Autodesk Inventor part; units mm, degrees
ref_plane "YZ Plane" through (0, 0, 0) normal (1, 0, 0) x (0, 1, 0)
ref_plane "XZ Plane" through (0, 0, 0) normal (0, 1, 0) x (-1, 0, 0)
ref_plane "XY Plane" through (0, 0, 0) normal (0, 0, 1) x (1, 0, 0)
sketch "Skizze1" plane through (0, 0, 0) normal (0, 0, 1) x (1, 0, 0)
  line L0 (15, -9.5) -> (-15, -9.5)
  line L1 (-15, -9.5) -> (-15, 9.5)
  line L2 (-15, 9.5) -> (15, 9.5)
  line L3 (15, 9.5) -> (15, -9.5)
  line L4 (15, -9.5) -> (-15, 9.5) construction
  line L5 (-15, -9.5) -> (15, 9.5) construction
  point P0 (0, 0)
  dimension "d0" = 30
  dimension "d1" = 19
extrude "Extrusion1" add sketch "Skizze1" along normal blind 22
sketch "Skizze7" plane through (0, 0, 22) normal (0, 0, 1) x (1, 0, 0)
  line L0 (-7.5, -7.5) -> (-7.5, 7.5)
  line L1 (-7.5, 7.5) -> (7.5, 7.5)
  line L2 (7.5, 7.5) -> (7.5, -7.5)
  line L3 (7.5, -7.5) -> (-7.5, -7.5)
  line L4 (15, -9.5) -> (15, 9.5)
  point P0 (0, 0)
  point P1 (0, -7.5)
  point P2 (7.5, 0)
  point P3 (15, 0)
  dimension "d36" = 15
  dimension "d37" = 15
extrude "Extrusion3" add sketch "Skizze7" along normal blind 60
chamfer "Fasen1" distance 2.5 angle 45 2 edges at (-7.5, 7.5, 52) (7.5, 7.5, 52)
sketch "Skizze2" plane through (-15, -9.5, 22) normal (0, 0, 1) x (1, 0, 0)
  line L0 (7, 17.25) -> (23, 17.25)
  line L1 (23, 17.25) -> (23, 1.75)
  line L2 (23, 1.75) -> (7, 1.75)
  line L3 (7, 1.75) -> (7, 17.25)
  line L4 (0, 0) -> (30, 0)
  point P0 (15, 9.5)
  point P1 (15, 1.75)
  point P2 (15, 0)
  point P3 (7, 9.5)
  dimension "d4" = 16
  dimension "d7" = 15.5
extrude "Extrusion2" add sketch "Skizze2" along normal blind 55
sketch "Skizze3" plane through (-15, -9.5, 82) normal (0, 0, 1) x (1, 0, 0)
  line L0 (23, 1.75) -> (23, 17.25)
  line L1 (23, 17.25) -> (7, 17.25)
  point P0 (15, 9.5)
  point P1 (15, 9.5)
  point P2 (23, 9.5)
  point P3 (15, 17.25)
hole "Bohrung1" at (0, 0, 82) direction (0, 0, -1) diameter 2.459 depth 15 tip angle 118
sketch "Skizze4" plane through (-15, -9.5, 0) normal (0, -1, 0) x (1, 0, 0)
  line L0 (0, 0) -> (30, 0)
  line L1 (7, 77) -> (23, 77)
  line L2 (7.5, 82) -> (22.5, 82)
  point P0 (15, 0)
  point P1 (15, 9)
  point P2 (15, 0)
  dimension "d43" = 73
hole "Bohrung2" at (0, -9.5, 9) direction (0, 1, 0) diameter 7.5 depth 9.5 counterbore diameter 10 counterbore depth 4
mirror "Spiegeln1" about plane through (0, 0, 0) normal (0, 1, 0) of "Bohrung2"
sketch "Skizze5" plane through (0, 0, 22) normal (0, 0, 1) x (1, 0, 0)
  circle A0 centre (0, 0) radius 1.2295
  line L0 (15, 9.5) -> (-15, 9.5)
  line L1 (-15, -9.5) -> (15, -9.5)
  point P0 (12, -3)
  point P1 (-12, -3)
  dimension "d30" = 24
  dimension "d31" = 12
  dimension "d34" = 6.5
  dimension "d35" = 6.5
hole "Bohrung3" at (12, -3, 22) at (-12, -3, 22) direction (0, 0, -1) diameter 3.1 depth 22
properties part number "Lagerbock" material "Stahl, galvanisiert"
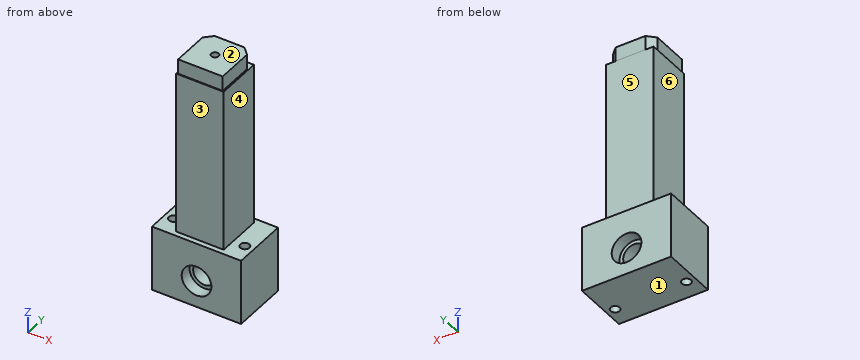
Geometry check sheet. Reference: the model listing, model coordinates, mm. Face numbers are marked on the shaded views. A direction names the side the tool comes from. Give positions to 0.01 mm unless a question says otherwise; leave off trailing zeros. Order: outer loops, then holes, each group sorted by start corner. A loop starts at its lowest first (then second) coordinate and runs counter-clockwise, first axis right, second up.
1. Section check D-D, the plane z = 11.5. Enter the section's corners in (x, y), and give its area (3 significant figures).
2. Access from +Z, -Z, +X, -X, +Y, -Y to the whole of each face (thin tool, end or side, straight path). Record for the marked faces 4, 5 and 6.
3. Section check C-C, the plane z = 74.5. Enter the section's corners in (x, y), and give its area (3 significant figures).
4. Section check A-A, the plane y = -6.75. Enter the section's corners in (x, z).
5. Thickness scan on L1, parallel to X at y = -3, z = 13; L2, parallel to X at y = -3, z = 8.75; L3, parallel to Z at x = 0, y = 6.55. Record the ranges inside material, lowest first.
6. Gauge pin test, flat ends, axial feed: pin 1 Ø8 at (y, z) = (0, 46) entering from -X; pin 2 Ø1.5 at (y, z) = (0.5, 80.5) entering from -X; pin 3 Ø5.5 at (x, z) = (0.5, 80.5) entering from +Y. Record the tip position at first contact, or that the pin passes through.
7. Release check for a two-part mould opening along Z. For the marked faces 1, 2 and 3 record: pulls with the +Z half, pulls with the -Z half, needs draft (parallel to the pull), parting line crosses it, or undercut.
8. Section check B-B, the plane x = 12. Enter the section's corners in (y, z), and give its area (3 significant figures).
Values follow:
1. outline: (-15, -9.5) - (-4.33, -9.5) - (-4.33, -5.5) - (-2.8, -5.5) - (-2.8, 5.5) - (-4.33, 5.5) - (-4.33, 9.5) - (-15, 9.5) - close; (2.8, -5.5) - (4.33, -5.5) - (4.33, -9.5) - (15, -9.5) - (15, 9.5) - (4.33, 9.5) - (4.33, 5.5) - (2.8, 5.5) - close; hole circle Ø3.1 at (-12, -3); hole circle Ø3.1 at (12, -3)
1. area: 424 mm2
2. face 4: +Z, +X, +Y, -Y
2. face 5: +Z, +X, -X, +Y
2. face 6: +Z, -X, +Y, -Y
3. outline: (-8, -7.75) - (8, -7.75) - (8, 7.75) - (-8, 7.75) - close; hole circle Ø2.46 at (0, 0)
3. area: 243 mm2
4. outline: (-15, 0) - (15, 0) - (15, 22) - (8, 22) - (8, 77) - (7.5, 77) - (7.5, 82) - (-7.5, 82) - (-7.5, 77) - (-8, 77) - (-8, 22) - (-15, 22) - close; hole circle Ø10 at (0, 9)
5. L1: x = -15 to -13.55, -10.45 to 10.45, 13.55 to 15
5. L2: x = -15 to -13.55, -10.45 to -3.74, 3.74 to 10.45, 13.55 to 15
5. L3: z = 0 to 4, 14 to 82
6. pin 1: stops at x = -8
6. pin 2: stops at x = -7.5
6. pin 3: stops at y = 7.5
7. face 1: pulls with the -Z half
7. face 2: pulls with the +Z half
7. face 3: needs draft
8. outline: (-9.5, 0) - (-4.55, 0) - (-4.55, 22) - (-9.5, 22) - close; (-1.45, 0) - (9.5, 0) - (9.5, 22) - (-1.45, 22) - close
8. area: 350 mm2
